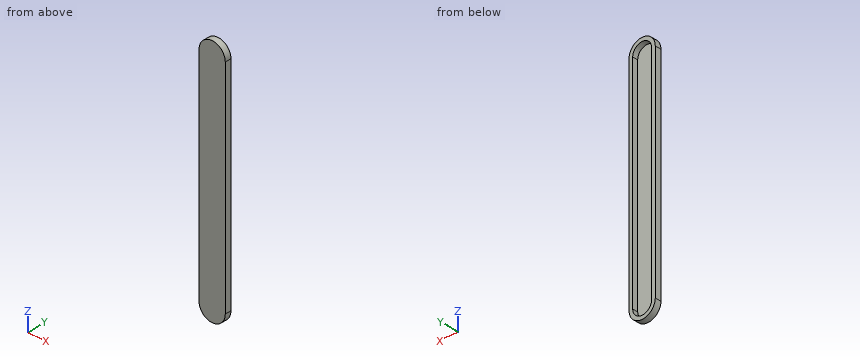
Autodesk Inventor part; units mm, degrees
ref_plane "YZ Plane" through (0, 0, 0) normal (1, 0, 0) x (0, 1, 0)
ref_plane "XZ Plane" through (0, 0, 0) normal (0, 1, 0) x (-1, 0, 0)
ref_plane "XY Plane" through (0, 0, 0) normal (0, 0, 1) x (1, 0, 0)
ref_plane "Work Plane1" through (-54.4323, -35.9721, 73.855) normal (0, 1, 0) x (-1, 0, 0)
sketch "Sketch1" plane through (-54.4323, -35.9721, 73.855) normal (0, 1, 0) x (-1, 0, 0)
  arc A0 (7.2, 60.25) -> (-7.2, 60.25) centre (0, 60.25) ccw
  line L0 (-7.2, -60.25) -> (-7.2, 60.25)
  arc A1 (-7.2, -60.25) -> (7.2, -60.25) centre (0, -60.25) ccw
  line L1 (7.2, 60.25) -> (7.2, -60.25)
  arc A2 (-5.2, -60.25) -> (5.2, -60.25) centre (0, -60.25) ccw
  line L2 (-5.2, -60.25) -> (-5.2, 60.25)
  line L3 (5.2, 60.25) -> (5.2, -60.25)
  arc A3 (5.2, 60.25) -> (-5.2, 60.25) centre (0, 60.25) ccw
  point P0 (-54.4323, -73.855)
extrude "Extrusion1" add sketch "Sketch1" along normal blind 0.4 contours L1 A1 L0 A0 | L2 A3 L3 A2
sketch "Sketch2" plane through (-54.4323, -35.5721, 73.855) normal (0, 1, 0) x (1, 0, 0)
  arc A0 (-7.2, -60.25) -> (7.2, -60.25) centre (0, -60.25) ccw
  line L0 (-7.2, -60.25) -> (-7.2, 60.25)
  arc A1 (7.2, 60.25) -> (-7.2, 60.25) centre (0, 60.25) ccw
  line L1 (7.2, 60.25) -> (7.2, -60.25)
  line L2 (5.2, -60.25) -> (5.2, 60.25)
  arc A2 (5.2, 60.25) -> (-5.2, 60.25) centre (0, 60.25) ccw
  line L3 (-5.2, 60.25) -> (-5.2, -60.25)
  arc A3 (-5.2, -60.25) -> (5.2, -60.25) centre (0, -60.25) ccw
  point P0 (54.4323, 73.855)
extrude "Extrusion2" add sketch "Sketch2" along normal blind 3
properties part number "wiper_outside" material "ABS Plastic"
Here's how the part is built. I have some questions about the finished solid (model axes, mm). Give positions to 0.01 mm unless a question says otherwise; leave off trailing zeros. Loops run counter-clockwise (first coordinate to the right, second up) from the corner with the lowest first, then second, coordinate; pieces in that order, holes last. Notation, with made-up numbers: M 12,-31.5 L 54,-31.5 A24 cw 54,-15.5 Z; hole C 1.25,34.5 d7. An arc over 180 degrees is marked long. Put each result on its own line as item: value. Start each with the question number.
(1) I need wall thicknesses on line 1 along Z through (x, y) = (-54.75, -32.75); line 2 along X through (y, z) = (-34.75, 101.5); line 3 along Y through (x, z) = (-51.25, 82.5). Which ranges of each line are inside material? Lowest first, please. Write a range as [from, to].
(2) I want a section at B-B on y = -34.9. Please give me the cut outline in (x, z) (3 decimals), then the cut area to 3 significant figures.
(3) Will these pins go through, and if not, where does the flat tip stop? pin 1 Ø3 at (x, z) = (-57, 45) entering from +Y; pin 2 Ø1.5 at (x, y) = (-55.5, -33.5) entering from -Z.
(4) I want a section at A-A on z = 68.5. Please give me the cut outline in (x, y).
(5) I want a section at C-C on x = -51.5. Please give me the cut outline in (y, z).
Answer block:
1. line 1: [6.41, 8.41], [139.3, 141.3]
1. line 2: [-61.63, -59.63], [-49.23, -47.23]
1. line 3: [-35.97, -35.57]
2. outline: M -61.632,13.605 A7.2 ccw -47.232,13.605 L -47.232,134.105 A7.2 ccw -61.632,134.105 Z; hole M -59.632,13.605 A5.2 ccw -49.232,13.605 L -49.232,134.105 A5.2 ccw -59.632,134.105 Z
2. area: 560 mm^2
3. pin 1: y = -35.57
3. pin 2: z = 6.41
4. outline: M -61.63,-35.97 L -47.23,-35.97 L -47.23,-32.57 L -49.23,-32.57 L -49.23,-35.57 L -59.63,-35.57 L -59.63,-32.57 L -61.63,-32.57 Z
5. outline: M -35.97,7.03 L -32.57,7.03 L -32.57,9.31 L -35.57,9.31 L -35.57,138.4 L -32.57,138.4 L -32.57,140.68 L -35.97,140.68 Z
